Can you work these out from the model? Positions are in its coordinate system, mm. A direction names the side the tool comes from. Round coordinates to 2 decimals unless told otherwise and drop trailing zeros. Order: outer loops, then holes, each group sorted by start corner. A loop starts at its lowest first (then second) coordinate and runs counter-clockwise, first axis right, second up. Notation, with made-up numbers: (-19.5, 24) -> (4.5, 24) arc R20 ccw to (4.5, 59) -> close; hole circle Ø9 at (88, 53). An arc over 180 degrees is marked (long way). Use a Markdown table: item, result. Add a question column.
Q1. If we section it at B-B on y = 32: List the corners of the cut face in (x, z) for me.
Q2. If we section it at D-D on x = 48: List the corners of the cut face in (y, z) for me, plus the area to 3 significant figures.
Q3. I need wall thicknesses on line 1 along Y through (x, z) = (97, 0.6); line 2 along X through (y, z) = (48, 1.65); line 3 along Z through (x, y) = (46, 21.5). Which ranges of each line are inside material? Lowest first, please. Write a range as [from, to].
Q4. I'm going to push flat-ended pins straight in: pin 1 Ø0.5 at (y, z) = (43.5, 2.5) entering from -X; pin 2 Ø3 at (x, y) = (97, 3) entering from +Z; pin 3 Ø0.8 at (x, z) = (25.5, 2.5) entering from +Y; pin 4 Ø2.5 at (x, y) = (97, 47) entering from -Z. Where does each tip first touch, or does it pass through?
Q5. If we section it at C-C on x = 62.5: List the corners of the cut face in (y, z) for me.
Q6. If we section it at A-A on x = 29: List the corners of the cut face in (y, z) for me, plus the area to 3 significant figures.
Q7. We'd pull the mould along Y, two halves only. Please class faces 6 (the face through (49, 50, 1)), 7 (the face through (0, 25, 1)), 8 (the face through (95.9, 3, 1)): +Y half, -Y half, draft (parallel to the pull), parting line (faces both ways), or undercut.
Q8. For faces 1 (the face through (94.49, 44.65, 2.49)), 2 (the face through (5.51, 44.65, 2.49)), 3 (the face through (94.65, 5.51, 2.49)), 4 (the face through (57, 24.8, 2.5)), 5 (the face through (5.35, 5.51, 2.49)), which set-ups out of +Z, -Z, +X, -X, +Y, -Y let a thin tool reach every point of the face, with its end or its side?
```python
from build123d import *

# Parameters (mm, degrees)
ESQUISSE1_W        = 100
ESQUISSE1_H        = 50
ESQUISSE1_R        = 1.1
BOSS_EXTRU_1_DEPTH = 2
BOSS_EXTRU_2_DEPTH = 1


with BuildPart() as part:
    # Esquisse1 → Boss.-Extru.1 (new body)
    with BuildSketch(Plane.XY):
        with Locations((50, 25)):
            Rectangle(ESQUISSE1_W, ESQUISSE1_H)
        with Locations((3, 47)):
            Circle(ESQUISSE1_R, mode=Mode.SUBTRACT)
        with Locations((97, 47)):
            Circle(ESQUISSE1_R, mode=Mode.SUBTRACT)
        with Locations((3, 3)):
            Circle(ESQUISSE1_R, mode=Mode.SUBTRACT)
        with Locations((97, 3)):
            Circle(ESQUISSE1_R, mode=Mode.SUBTRACT)
    extrude(amount=BOSS_EXTRU_1_DEPTH)

    # Esquisse2 → Boss.-Extru.2 (add)
    with BuildSketch(Plane.XY.offset(2)):
        with BuildLine():
            Line((2.5, 37.5), (2.5, 12.5))
            ThreePointArc((2.5, 12.5), (5.428932188, 5.428932188), (12.5, 2.5))
            Line((12.5, 2.5), (35.5, 2.5))
            Line((35.5, 2.5), (35.5, 10.379808483))
            ThreePointArc((35.5, 10.379808483), (43, 25), (35.5, 39.620191517))
            Line((35.5, 39.620191517), (35.5, 47.5))
            Line((35.5, 47.5), (12.5, 47.5))
            ThreePointArc((12.5, 47.5), (5.428932188, 44.571067812), (2.5, 37.5))
        make_face()
        with BuildLine():
            Line((64.5, 39.620191517), (64.5, 47.5))
            Line((64.5, 47.5), (87.5, 47.5))
            ThreePointArc((87.5, 47.5), (94.571067812, 44.571067812), (97.5, 37.5))
            Line((97.5, 37.5), (97.5, 12.5))
            ThreePointArc((97.5, 12.5), (94.571067812, 5.428932188), (87.5, 2.5))
            Line((87.5, 2.5), (64.5, 2.5))
            Line((64.5, 2.5), (64.5, 10.379808483))
            ThreePointArc((64.5, 10.379808483), (57, 25), (64.5, 39.620191517))
        make_face()
    extrude(amount=BOSS_EXTRU_2_DEPTH)


solid = part.part
```
Answer below:
| question | item | result |
|---|---|---|
| 1 | outline | (0, 0) -> (100, 0) -> (100, 2) -> (97.5, 2) -> (97.5, 3) -> (58.42, 3) -> (58.42, 2) -> (41.58, 2) -> (41.58, 3) -> (2.5, 3) -> (2.5, 2) -> (0, 2) -> close |
| 2 | outline | (0, 0) -> (50, 0) -> (50, 2) -> (0, 2) -> close |
| 2 | area | 100 mm² |
| 3 | line 1 | [0, 1.9], [4.1, 45.9], [48.1, 50] |
| 3 | line 2 | [0, 2.54], [3.46, 96.54], [97.46, 100] |
| 3 | line 3 | [0, 2] |
| 4 | pin 1 | x = 4.32 |
| 4 | pin 2 | z = 2 |
| 4 | pin 3 | y = 47.5 |
| 4 | pin 4 | z = 0 |
| 5 | outline | (0, 0) -> (50, 0) -> (50, 2) -> (37.95, 2) -> (37.95, 3) -> (12.05, 3) -> (12.05, 2) -> (0, 2) -> close |
| 6 | outline | (0, 0) -> (50, 0) -> (50, 2) -> (47.5, 2) -> (47.5, 3) -> (2.5, 3) -> (2.5, 2) -> (0, 2) -> close |
| 6 | area | 145 mm² |
| 7 | face 6 | +Y half |
| 7 | face 7 | draft |
| 7 | face 8 | undercut |
| 8 | face 1 | +Z, +X, +Y |
| 8 | face 2 | +Z, -X, +Y |
| 8 | face 3 | +Z, +X, -Y |
| 8 | face 4 | +Z |
| 8 | face 5 | +Z, -X, -Y |
